Geometry: final body of the model. Coordinates: model frame, mm. Face numbers are marked on the shaded views. A direction names the side the tool comes from. Give positions to 0.01 mm unless a question says otherwise; leave off trailing zeros. Write each loop counter-clockwise with the first axis right and the second up, starting at its lowest first coordinate (ties: lowest second). Pieces come first, ordered by that corner, then holes. Notation, with made-up numbers: (74.5, 41.5) -> (120.5, 41.5) arc R30 ccw to (120.5, 76.5) -> close; hole circle Ø9 at (5.25, 39.25). An arc over 180 degrees is marked (long way). Answer in a Markdown table with one row per item. Add a question column.
Item 1: Section query D-D on z = -103.5. Output: boundary loops of the cut face in (x, y), plus the area to 3 significant figures.
Item 2: Access query for the marked faces 1 and 2. Directions: +Z, -Z, +X, -X, +Y, -Y. A direction counts if a zero-diameter tool reaches every point of the face in a straight line with its end or side. Return the directions, or none.
Item 3: Section query B-B on z = -84. Output: boundary loops of the cut face in (x, y), plus the area to 3 significant figures.
Item 4: Section query C-C on y = -195. Output: boundary loops of the cut face in (x, z).
Item 5: Material intervals for probe 1 along Y at (x, z) = (-46, -40); probe 2 along X at (y, z) = (-14, -17.5); probe 3 along X at (y, z) = (-26, -58), sorted ascending. Write a range as from..to.
Item 6: First-contact query: P1, Ø3, axis at x = 23, z = -95, coming from the +Y side; P2, Ø1, axis at y = -103, z = -50.5, coming from the -X side; P3, Ø1.5, axis at y = -42, z = -25.5, coming from the +X side; P4, Ø12, axis at x = -7.5, y = -95.5, coming from the +Z side. Flat tips, straight axial feed; report the tip coordinate or a pass-through.
Item 7: Section query A-A on x = 0. Output: boundary loops of the cut face in (y, z).
```python
from build123d import *

# Parameters (mm, degrees)
F0_R     = 125
F1_DEPTH = 300
F3_T     = -2.5
F5_DEPTH = 331


with BuildPart() as f1:
    # F0 (on Front) → F1 (new body)
    with BuildSketch(Plane.XZ):
        Circle(F0_R)
    extrude(amount=F1_DEPTH)

    # F3
    f3_openings = [f1.faces().sort_by_distance(p)[0] for p in [
        (0, -300, 0),
    ]]
    offset(amount=F3_T, openings=f3_openings)

    # F4 (on offset) → F5 (cut)
    with BuildSketch(Plane.YZ.offset(125)):
        with BuildLine():
            Line((-278.461281, -65.740379), (0, 0))
            Line((0, 0), (37.560482, 139.173388))
            Line((37.560482, 139.173388), (-357.278258, 144.254044))
            Line((-357.278258, 144.254044), (-367.802441, -101.419425))
            Line((-367.802441, -101.419425), (-308.549038, -101.419425))
            ThreePointArc((-308.549038, -101.419425), (-299.400873, -78.60811), (-278.461281, -65.740379))
        make_face()
    extrude(amount=-F5_DEPTH, mode=Mode.SUBTRACT)


solid = f1.part
```
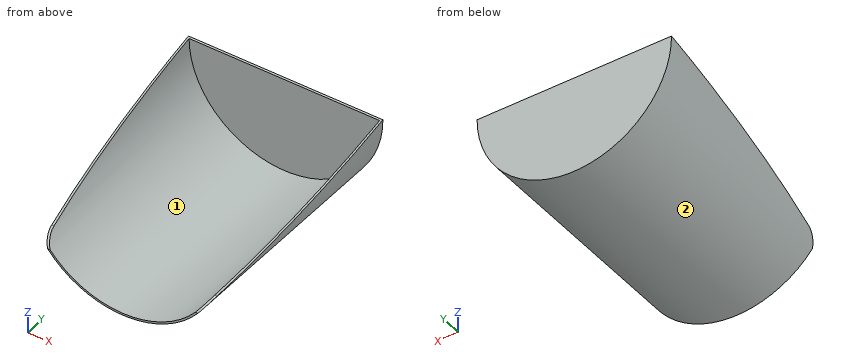
Findings below:
| question | item | result |
|---|---|---|
| 1 | outline | (-70.09, -300) -> (-65.53, -300) -> (-65.53, -2.5) -> (65.53, -2.5) -> (65.53, -300) -> (70.09, -300) -> (70.09, 0) -> (-70.09, 0) -> close |
| 1 | area | 3,070 mm^2 |
| 2 | face 1 | +Z, -Y |
| 2 | face 2 | -Z, +Y, -Y |
| 3 | outline | (-92.57, -300) -> (-89.16, -300) -> (-89.16, -2.5) -> (89.16, -2.5) -> (89.16, -300) -> (92.57, -300) -> (92.57, 0) -> (-92.57, 0) -> close |
| 3 | area | 2,490 mm^2 |
| 4 | outline | (-116.21, -46.04) arc R125 ccw to (116.21, -46.04) -> (113.52, -46.04) arc R122.5 cw to (-113.52, -46.04) -> close |
| 5 | probe 1 | y = -2.5..0 |
| 5 | probe 2 | x = -123.77..-121.24, 121.24..123.77 |
| 5 | probe 3 | x = -110.73..-107.9, 107.9..110.73 |
| 6 | P1 | stops at y = 0 |
| 6 | P2 | stops at x = -114.56 |
| 6 | P3 | stops at x = 122.53 |
| 6 | P4 | stops at z = -121.75 |
| 7 | outline | (-300, -125) -> (0, -125) -> (0, 0) -> (-2.5, -0.59) -> (-2.5, -122.5) -> (-300, -122.5) -> close |
